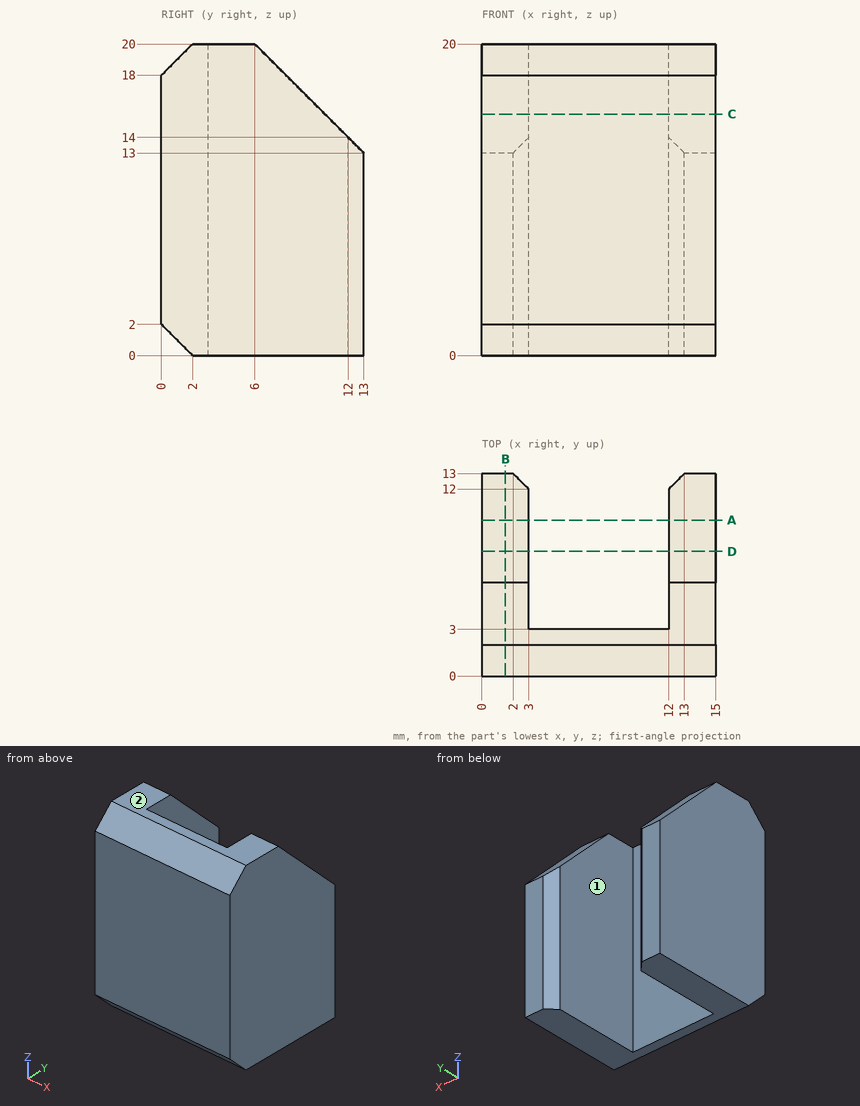
Source: three-view drawing plus pictorial views. Frame: mm from the lowest corner of the part. A direction names the side the tool comes from. Round coordinates to 2 decimals unless told otherwise and drop trailing zeros. Loops run counter-clockwise (first coordinate to the right, second up) from the corner with the lowest first, then second, coordinate; pieces in that order, holes last.
Q1. Section A-A on y = 10. Return loops of the section in (x, z), plus the area to 3 significant figures.
Q2. Section C-C on z = 15.5. Return loops of the section in (x, y), plus the area to 3 significant figures.
Q3. Section B-B on x = 1.5. Return loops of the section in (y, z).
Q4. Section D-D on y = 8. Return loops of the section in (x, z), plus the area to 3 significant figures.
Q5. Access query for the marked faces 1 and 2. Directions: +Z, -Z, +X, -X, +Y, -Y. A direction counts if a zero-diameter tool reaches every point of the face in a straight line with its end or side. Return the directions, or none.
Q6. Material intervals for L1, parallel to X at y = 11.25, z = 13; L2, parallel to Y at x = 6, z = 14.25; L3, parallel to Z at x = 2.75, y = 12, sorted ascending.
Q7. Pin query (flat end, axial travel): P1, Ø4, axis at x = 7, z = 3.5, coming from the +Y side. Return the tip coordinate at first contact, or that it passes through.
Evaluation:
1. outline: (0, 0) - (3, 0) - (3, 16) - (0, 16) - close; (12, 0) - (15, 0) - (15, 16) - (12, 16) - close
1. area: 96.0 mm2
2. outline: (0, 0) - (15, 0) - (15, 10.5) - (12, 10.5) - (12, 3) - (3, 3) - (3, 10.5) - (0, 10.5) - close
2. area: 90.0 mm2
3. outline: (0, 2) - (2, 0) - (13, 0) - (13, 13) - (6, 20) - (2, 20) - (0, 18) - close
4. outline: (0, 0) - (3, 0) - (3, 18) - (0, 18) - close; (12, 0) - (15, 0) - (15, 18) - (12, 18) - close
4. area: 108 mm2
5. face 1: +Z, -Z, +Y
5. face 2: +Z, +X, -X, +Y, -Y
6. L1: x = 0 to 3, 12 to 15
6. L2: y = 0 to 3
6. L3: z = 0 to 14
7. P1: stops at y = 3
